Verification items for this drawing (mm, ordinates from the low corner). Coordinates: 2 decimals unless noted, no trailing zeros. Loops run counter-clockwise (first coordinate to the right, second up) from the corner with the lowest first, then second, coordinate; pieces in that order, holes last. Notation, with made-up numbers: (-1, -13) -> (38, -13) arc R25 cw to (38, 6) -> close; hole circle Ø11 at (10.25, 24). An arc over 180 degrees is marked (long way). Write item = value, one per line.
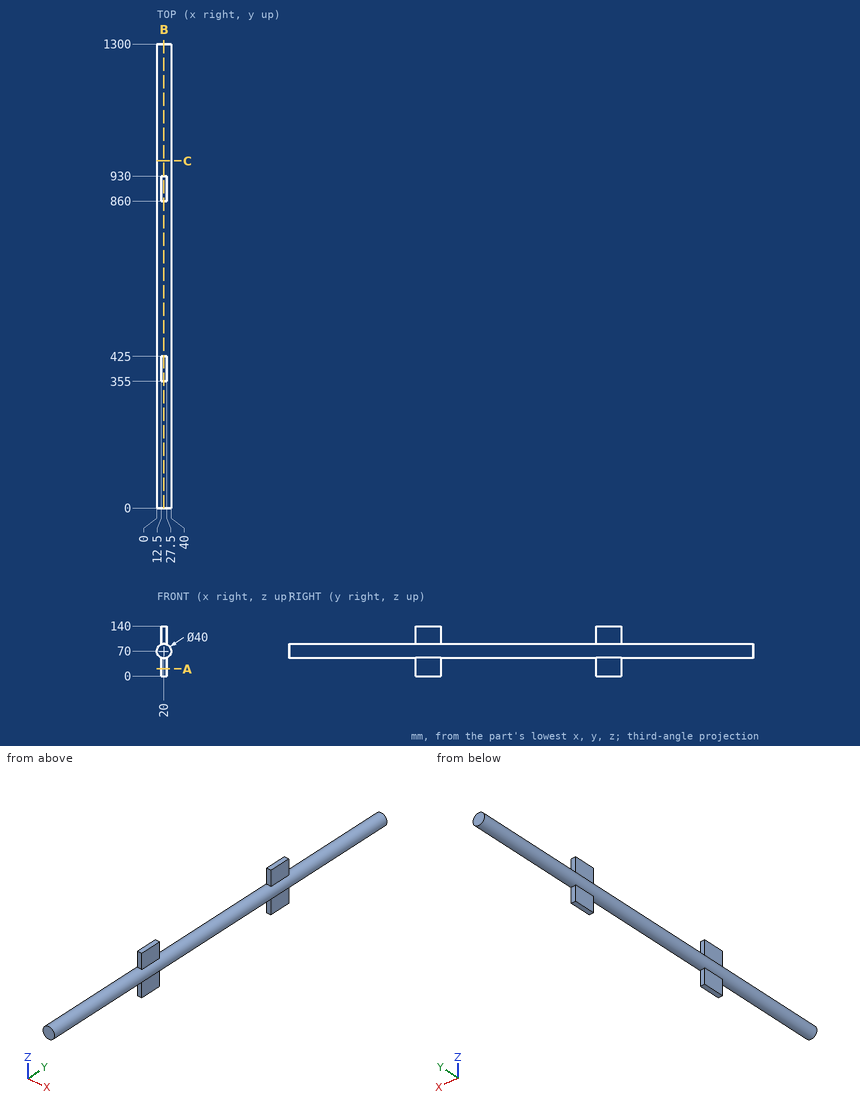
1) Depth check by flat-ended pin: pin 1 Ø16.5 at (x, z) = (18, 103.5) entering from +Y; pin 2 Ø16.5 at (x, z) = (19, 37) entering from -Y; pin 3 Ø12 at (y, z) = (1157.5, 71.5) entering from -X; pin 4 Ø2 at (x, z) = (4, 81.5) entering from -Y. Enter the tip coordinate at first touch or a pass-through.
Ans:
pin_1 = 930
pin_2 = 355
pin_3 = 0
pin_4 = 0
2) Sectioned sample at A-A, the plane z = 20. Record the cut outline in (x, y), plus the area to 3 significant figures.
Ans:
outline = (12.5, 355) -> (27.5, 355) -> (27.5, 425) -> (12.5, 425) -> close; (12.5, 860) -> (27.5, 860) -> (27.5, 930) -> (12.5, 930) -> close
area = 2,100 mm2
3) Sectioned sample at B-B, the plane x = 20. Record the cut outline in (y, z).
Ans:
outline = (0, 50) -> (355, 50) -> (355, 0) -> (425, 0) -> (425, 50) -> (860, 50) -> (860, 0) -> (930, 0) -> (930, 50) -> (1300, 50) -> (1300, 90) -> (930, 90) -> (930, 140) -> (860, 140) -> (860, 90) -> (425, 90) -> (425, 140) -> (355, 140) -> (355, 90) -> (0, 90) -> close
4) Sectioned sample at C-C, the plane y = 972.5. Record the cut outline in (x, z), plus the area to 3 significant figures.
Ans:
outline = circle Ø40 at (20, 70)
area = 1,260 mm2
5) Material ranges on line 1 (Y direction, x = 19, z = 8); line 2 (Z direction, x = 21.5, y = 208); line 3 (Z direction, x = 19, y = 1158.5), recorded low to high.
Ans:
line_1 = 355 to 425, 860 to 930
line_2 = 50.06 to 89.94
line_3 = 50.03 to 89.97
